Answer from the drawing. Dimensions are ordinates in mm from the lowest x, y and z of the part. A direction names the side the tool comes from. Round coordinates to 2 decimals unless told otherwise and drop trailing zeros. Loops run counter-clockwise (first coordinate to the right, second up) from the corner with the lowest first, then second, coordinate; pieces in that order, holes last. Notation, with made-up numbers: (57.25, 87) - (115.25, 87) arc R36 cw to (115.25, 124) - close; hole circle Ø3 at (53, 60). An arc over 180 degrees is marked (long way). Answer as CSV lines item,"result". Start each with the question number.
Q1. Section A-A on y = 13.5 is taken. Write down the section's boundary in (x, z) (3 decimals).
Q2. Each of these flat-tipped pins is pushed along its axis until it touches: pin 1 Ø12 at (x, z) = (9.5, 85) entering from +Y; pin 2 Ø4 at (x, y) = (3.5, 22.5) entering from -Z; pin 3 Ø12 at (x, y) = (15.5, 7.5) entering from +Z; pin 4 Ø1.5 at (x, y) = (4.5, 17) entering from +Z. Where does it stop, or does it pass through?
Q3. Section D-D on z = 90 is taken. Write down the section's boundary in (x, y) (3 decimals), then the cut area to 3 significant figures.
Q4. Section B-B on x = 6.5 is taken. Write down the section's boundary in (y, z) (3 decimals), then the cut area to 3 significant figures.
Q5. The mould has two halves that part along Y. Classify the marked faces 1, 2 and 3: +Y half, -Y half, draft (parallel to the pull), parting line (faces both ways), or undercut.
Q6. For the marked faces 4 and 5, determine the directions among +Z, -Z, +X, -X, +Y, -Y from which every point of the face is accessible in a straight line to the end or side of a thin tool.
Q7. Section C-C on z = 46 is taken. Write down the section's boundary in (x, y) (3 decimals), then the cut area to 3 significant figures.
Q8. Straight lines are drawn through the part: L1, parallel to Y at x = 12.75, z = 51 (3 decimals); L2, parallel to Y at x = 16, z = 85 (3 decimals). For each, find the intervals that lie inside material, in ascending order. Write a range as [from, to].
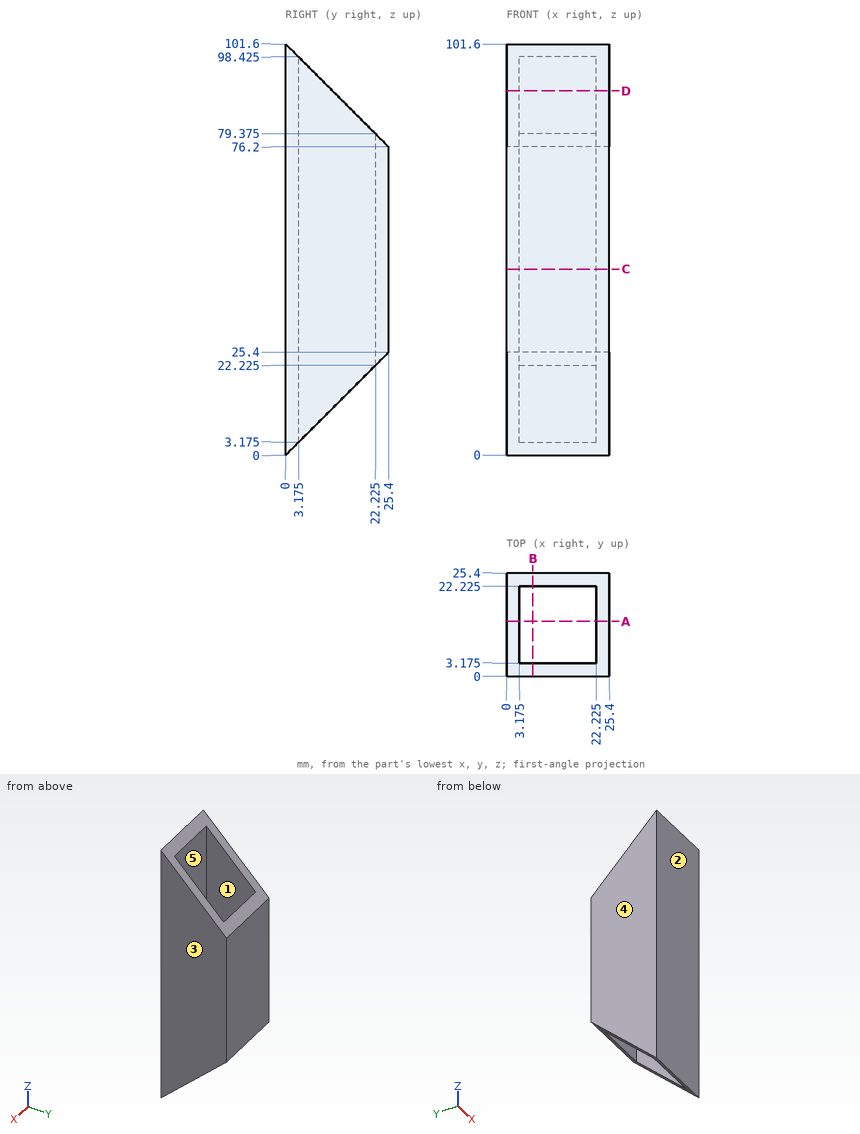
Findings:
1,outline,"(0, 13.5) - (3.175, 13.5) - (3.175, 88.1) - (0, 88.1) - close; (22.225, 13.5) - (25.4, 13.5) - (25.4, 88.1) - (22.225, 88.1) - close"
2,pin 1,"stops at y = 22.6"
2,pin 2,"stops at z = 20.53"
2,pin 3,"stops at z = 100.1"
2,pin 4,"passes through"
3,outline,"(0, 0) - (25.4, 0) - (25.4, 11.6) - (22.225, 11.6) - (22.225, 3.175) - (3.175, 3.175) - (3.175, 11.6) - (0, 11.6) - close"
3,area,"134 mm^2"
4,outline,"(0, 0) - (3.175, 3.175) - (3.175, 98.425) - (0, 101.6) - close; (22.225, 22.225) - (25.4, 25.4) - (25.4, 76.2) - (22.225, 79.375) - close"
4,area,"484 mm^2"
5,face 1,"undercut"
5,face 2,"-Y half"
5,face 3,"draft"
6,face 4,"+Z, -Z, -X, +Y, -Y"
6,face 5,"+Z, -Z"
7,outline,"(0, 0) - (25.4, 0) - (25.4, 25.4) - (0, 25.4) - close; hole (3.175, 3.175) - (22.225, 3.175) - (22.225, 22.225) - (3.175, 22.225) - close"
7,area,"282 mm^2"
8,L1,"y = [0, 3.175], [22.225, 25.4]"
8,L2,"y = [0, 3.175]"
